```python
from build123d import *

# Parameters (mm, degrees)
SKETCH020_W     = 150
SKETCH020_H     = 100
PAD009_DEPTH    = 2.5
SKETCH005_W     = 140
SKETCH005_H     = 90
PAD010_DEPTH    = 2.5
SKETCH021_R     = 20
PAD002_DEPTH    = 50
SKETCH019_R     = 15
POCKET010_DEPTH = 50
SKETCH003_W     = 55
SKETCH003_H     = 70
POCKET001_DEPTH = 3
SKETCH004_R     = 1.5
POCKET002_DEPTH = 2.5
SKETCH006_W     = 28
SKETCH006_H     = 20
POCKET003_DEPTH = 2
SKETCH007_R     = 1.4
SKETCH007_W     = 10
SKETCH007_H     = 3
POCKET004_DEPTH = 50
FILLET_R        = 10


with BuildPart() as part:
    # Sketch020 → Pad009 (new body)
    with BuildSketch(Plane.XY):
        with Locations((75, 50)):
            Rectangle(SKETCH020_W, SKETCH020_H)
    extrude(amount=PAD009_DEPTH)

    # Sketch005 → Pad010 (join)
    with BuildSketch(Plane.XY):
        with Locations((75, 50)):
            Rectangle(SKETCH005_W, SKETCH005_H)
    extrude(amount=-PAD010_DEPTH)

    # Sketch021 → Pad002 (join)
    with BuildSketch(Plane.XY):
        with Locations((50, 50)):
            Circle(SKETCH021_R)
    extrude(amount=PAD002_DEPTH)

    # Sketch019 → Pocket010 (cut, symmetric)
    with BuildSketch(Plane.XY):
        with Locations((50, 50)):
            Circle(SKETCH019_R)
    extrude(amount=POCKET010_DEPTH, both=True, mode=Mode.SUBTRACT)

    # Sketch003 → Pocket001 (cut)
    with BuildSketch(Plane.XY):
        with Locations((112.5, 50)):
            Rectangle(SKETCH003_W, SKETCH003_H)
    extrude(amount=-POCKET001_DEPTH, mode=Mode.SUBTRACT)

    # Sketch004 → Pocket002 (cut, symmetric)
    with BuildSketch(Plane.XY):
        with Locations((121, 18.5)):
            Circle(SKETCH004_R)
        with Locations((136.5, 69)):
            Circle(SKETCH004_R)
        with Locations((93, 18.5)):
            Circle(SKETCH004_R)
    extrude(amount=POCKET002_DEPTH, both=True, mode=Mode.SUBTRACT)

    # Sketch006 → Pocket003 (cut)
    with BuildSketch(Plane.XY.offset(-2.5)):
        with Locations((52, 80)):
            Rectangle(SKETCH006_W, SKETCH006_H)
    extrude(amount=POCKET003_DEPTH, mode=Mode.SUBTRACT)

    # Sketch007 → Pocket004 (cut, symmetric)
    with BuildSketch(Plane.XY.offset(5.5)):
        with Locations((44.5, 88)):
            Circle(SKETCH007_R)
        with Locations((58.5, 88)):
            Circle(SKETCH007_R)
        with Locations((51.5, 92.5)):
            Rectangle(SKETCH007_W, SKETCH007_H)
    extrude(amount=POCKET004_DEPTH, both=True, mode=Mode.SUBTRACT)

    # Fillet
    fillet_edges = [part.edges().sort_by_distance(p)[0] for p in [
        (30, 50, 2.5),
    ]]
    fillet(fillet_edges, radius=FILLET_R)


solid = part.part
```
Design review of the part built by this model. Coordinates are the model's own, in mm. A direction names the side the tool comes from. Give positions to 0.01 mm unless a question says otherwise; leave off trailing zeros. Loops run counter-clockwise (first coordinate to the right, second up) from the corner with the lowest first, then second, coordinate; pieces in that order, holes last. Notation, with made-up numbers: M -27,12.5 L 6,12.5 A16 ccw 6,25.5 Z; hole C -20.75,7 d5. An arc over 180 degrees is marked long. Return JSON: item names as keys, results as strings. Group by question number.
Item 1: We need section B-B (x = 50). Give the boundary of the cut face in (y, z).
Item 2: Insertion check: pin 1 Ø0.6 at (x, z) = (47.5, -1.5) entering from +Y; pin 2 Ø1.6 at (x, z) = (47, -1.5) entering from -Y; pin 3 Ø12 at (x, z) = (55.5, 28) entering from -Y; pin 4 Ø1.2 at (y, z) = (55, -0.5) entering from -X. Each pin has a flat end and moves straight along its axis. Give the tip position at first contact, or say it passes through.
Item 3: We need section A-A (y = 50). Give the boundary of the cut face in (x, z), and give its area (3 significant figures).
Item 4: We need section C-C (z = 28.5). Give the boundary of the cut face in (x, y), and give its area (3 significant figures).
Item 5: Tool access review of faces 1 (the flat face through (51, 94, 0)), 2 (the flat face through (52, 80, -0.5)), 3 (the flat face through (53, 65, 50)): name each direction out of +Z, -Z, +X, -X, +Y, -Y from which nothing blocks a thin tool from reaching the whole face with its end or side.
Item 6: Mouldability with a two-part tool opening along Y and no side actions: class faces 4 (the flat face through (69, 2, 0)), 5 (the flat face through (56.5, 92, 0)), 6 (the cylindrical face through (69.076, 56.007, 30.988)) as released by +Y, released by -Y, zero draft, split by the parting line, or undercut.
Item 7: For probe 1 along X at (y, z) = (88, 1.75); probe 2 along Y at (x, z) = (44, 1); probe 3 along Y at (x, z) = (50, 35), list the stretches that pass through material, from the lowest coordinate up.
Output:
{
 "1": {"outline": "M 0,0 L 5,0 L 5,-2.5 L 35,-2.5 L 35,50 L 30,50 L 30,12.5 A10 cw 20,2.5 L 0,2.5 Z; M 65,-2.5 L 70,-2.5 L 70,-0.5 L 90,-0.5 L 90,-2.5 L 91,-2.5 L 91,2.5 L 80,2.5 A10 cw 70,12.5 L 70,50 L 65,50 Z; M 94,-2.5 L 95,-2.5 L 95,0 L 100,0 L 100,2.5 L 94,2.5 Z"},
 "2": {"pin 1": "stops at y = 95", "pin 2": "stops at y = 5", "pin 3": "stops at y = 30", "pin 4": "stops at x = 0"},
 "3": {"outline": "M 0,0 L 5,0 L 5,-2.5 L 35,-2.5 L 35,50 L 30,50 L 30,12.5 A10 cw 20,2.5 L 0,2.5 Z; M 65,-2.5 L 85,-2.5 L 85,0 L 140,0 L 140,-2.5 L 145,-2.5 L 145,0 L 150,0 L 150,2.5 L 80,2.5 A10 cw 70,12.5 L 70,50 L 65,50 Z", "area": "955 mm^2"},
 "4": {"outline": "C 50,50 d40; hole C 50,50 d30", "area": "550 mm^2"},
 "5": {"face 1": "+Z, -Z", "face 2": "-Z", "face 3": "+Z, +X, -X, +Y, -Y"},
 "6": {"face 4": "zero draft", "face 5": "undercut", "face 6": "split by the parting line"},
 "7": {"probe 1": "x = 0 to 43.1, 45.9 to 57.1, 59.9 to 150", "probe 2": "y = 0 to 36.25, 63.75 to 86.69, 89.31 to 100", "probe 3": "y = 30 to 35, 65 to 70"}
}
